from build123d import *

# Parameters (mm, degrees)
SKETCH1_W           = 62
SKETCH1_H           = 15
BOSS_EXTRUDE1_DEPTH = 3.2
CUT_EXTRUDE1_REACH  = 5.2
SKETCH2_R           = 2.625


with BuildPart() as part:
    # Sketch1 → Boss-Extrude1 (new body)
    with BuildSketch(Plane(origin=(0, 0, 0), x_dir=(1, 0, 0), z_dir=(0, 1, 0))):
        Rectangle(SKETCH1_W, SKETCH1_H)
    extrude(amount=BOSS_EXTRUDE1_DEPTH)

    # Sketch2 → Cut-Extrude1 (cut, up to next)
    with BuildSketch(Plane(origin=(0, 3.2, 0), x_dir=(1, 0, 0), z_dir=(0, 1, 0)), mode=Mode.PRIVATE) as cut_extrude1_sk1:
        with Locations((-18, 0)):
            Circle(SKETCH2_R)
    cut_extrude1_tool1 = extrude(cut_extrude1_sk1.sketch, amount=-CUT_EXTRUDE1_REACH, mode=Mode.PRIVATE) & part.part
    add(cut_extrude1_tool1.solids().sort_by_distance((-18, 3.2, 0))[0], mode=Mode.SUBTRACT)
    # Sketch2 → Cut-Extrude1 (cut, up to next)
    with BuildSketch(Plane(origin=(0, 3.2, 0), x_dir=(1, 0, 0), z_dir=(0, 1, 0)), mode=Mode.PRIVATE) as cut_extrude1_sk2:
        with Locations((18, 0)):
            Circle(SKETCH2_R)
    cut_extrude1_tool2 = extrude(cut_extrude1_sk2.sketch, amount=-CUT_EXTRUDE1_REACH, mode=Mode.PRIVATE) & part.part
    add(cut_extrude1_tool2.solids().sort_by_distance((18, 3.2, 0))[0], mode=Mode.SUBTRACT)


solid = part.part
For this review, take the finished solid that the model builds, in its own axes (mm). Round coordinates to 2 decimals unless told otherwise and drop trailing zeros. Write each loop counter-clockwise with the first axis right and the second up, starting at its lowest first coordinate (ties: lowest second). Pieces come first, ordered by that corner, then holes. Notation, with made-up numbers: (58, 0) -> (63, 0) arc R20 ccw to (63, 13) -> close; hole circle Ø4 at (62, 87). An arc over 180 degrees is marked (long way). Use CSV: the item, a comma, the result in double quotes.
(1) Consider section A-A, the plane z = 0. Give the boundary of the cut face in (x, y) (3 decimals).
Computed values:
outline,"(-31, 0) -> (-20.625, 0) -> (-20.625, 3.2) -> (-31, 3.2) -> close; (-15.375, 0) -> (15.375, 0) -> (15.375, 3.2) -> (-15.375, 3.2) -> close; (20.625, 0) -> (31, 0) -> (31, 3.2) -> (20.625, 3.2) -> close"
(2) Draft analysis for pull direction Z (two halves, no side actions). For faces 1 (the face through (0, 2, -7.5)), 2 (the face through (15.378, 1.622, -0.115)), 3 (the face through (0, 2, 7.5)), state which applies: +Z half, -Z half, draft (parallel to the pull), parting line (faces both ways), or undercut.
Computed values:
face 1,"-Z half"
face 2,"undercut"
face 3,"+Z half"
(3) Consider section B-B, the plane x = 18. Give the boundary of the cut face in (y, z) (3 decimals), plus the area to 3 significant figures.
Computed values:
outline,"(0, -7.5) -> (3.2, -7.5) -> (3.2, -2.625) -> (0, -2.625) -> close; (0, 2.625) -> (3.2, 2.625) -> (3.2, 7.5) -> (0, 7.5) -> close"
area,"31.2 mm²"
(4) Consider section C-C, the plane y = 2. Give the boundary of the cut face in (x, z) (3 decimals).
Computed values:
outline,"(-31, -7.5) -> (31, -7.5) -> (31, 7.5) -> (-31, 7.5) -> close; hole circle Ø5.25 at (-18, 0); hole circle Ø5.25 at (18, 0)"
(5) To check wall thickness, follow L1, parallel to X at y = 1.8, z = 0 (3 decimals); L2, parallel to Z at x = -18, y = 0.8 (3 decimals); L3, parallel to X at y = 2.8, z = -2.25. State the ranges of each line that lie inside material, in increasing order. Write a range as [from, to].
Computed values:
L1,"[-31, -20.625], [-15.375, 15.375], [20.625, 31]"
L2,"[-7.5, -2.625], [2.625, 7.5]"
L3,"[-31, -19.35], [-16.65, 16.65], [19.35, 31]"
(6) Clearance check with flat-ended pins moving along their axes: P1, Ø1, axis at x = 13.5, z = -6, coming from the -Y side; P2, Ø4.5, axis at x = 18, z = 0, coming from the -Y side. State where each tip first meets the part, or that it passes through.
Computed values:
P1,"y = 0"
P2,"through"
